```python
from build123d import *

# Parameters (mm, degrees)
SKETCH1_W               = 126
SKETCH1_H               = 126
BOSS_EXTRUDE1_DEPTH     = 5
SKETCH3_R               = 12.5
BOSS_EXTRUDE2_DEPTH     = 7.5
SKETCH4_R               = 3.45
CUT_EXTRUDE1_DEPTH      = 11.5
SKETCH6_R               = 3
CUT_EXTRUDE2_DEPTH      = 179.628805068
CHAMFER1_SIZE           = 10
CHAMFER1_SIZE_2         = 7.26542528
CUT_EXTRUDE3_DEPTH      = 179.348675353
CUT_EXTRUDE3_DEPTH_BACK = 179.348675353


with BuildPart() as part:
    # Sketch1 → Boss-Extrude1 (new body)
    with BuildSketch(Plane(origin=(0, 0, 0), x_dir=(1, 0, 0), z_dir=(0, 1, 0))):
        with Locations((63, 63)):
            Rectangle(SKETCH1_W, SKETCH1_H)
    extrude(amount=BOSS_EXTRUDE1_DEPTH)

    # Sketch3 → Boss-Extrude2 (add)
    with BuildSketch(Plane(origin=(0, 5, 0), x_dir=(1, 0, 0), z_dir=(0, 1, 0))):
        with Locations(Location((108.6, 108.6, 0), (0, 0, 90))):
            Circle(SKETCH3_R)
    extrude(amount=BOSS_EXTRUDE2_DEPTH)

    # Sketch4 → Cut-Extrude1 (cut)
    with BuildSketch(Plane.XZ):
        with Locations(Location((108.6, -108.6, 0), (0, 0, 270))):
            Circle(SKETCH4_R)
    extrude(amount=-CUT_EXTRUDE1_DEPTH, mode=Mode.SUBTRACT)

    # Sketch6 → Cut-Extrude2 (cut, through all)
    with BuildSketch(Plane(origin=(0, 12.5, 0), x_dir=(1, 0, 0), z_dir=(0, 1, 0))):
        with Locations(Location((108.6, 108.6, 0), (0, 0, 270))):
            Circle(SKETCH6_R)
    extrude(amount=-CUT_EXTRUDE2_DEPTH, mode=Mode.SUBTRACT)

    # Chamfer1
    # the kernel refuses this chamfer: 10, 7.26542528 mm, written as the material it takes off along each edge
    with BuildSketch(Plane(origin=(108.6, 12.5, -108.6), x_dir=(0, 0, -1), z_dir=(1, 0, 0))) as chamfer1_piece_1_section:
        Polygon((12.5, -CHAMFER1_SIZE), (12.5 - CHAMFER1_SIZE_2, 0), (12.5, 0), align=None)
    chamfer1_piece_1 = revolve(axis=Axis((108.6, 12.5, -108.6), (0, 1, 0)), mode=Mode.PRIVATE)
    chamfer1_piece_1 = split(chamfer1_piece_1, bisect_by=Plane(origin=(108.6, 5, -100.650989912), z_dir=(0, 1, 0)), keep=Keep.TOP, mode=Mode.PRIVATE)
    add(chamfer1_piece_1, mode=Mode.SUBTRACT)

    # Sketch7 → Cut-Extrude3 (cut, two sides: drawn at the far end of the back side and taken through both)
    with BuildSketch(Plane(origin=(0, 5, 0), x_dir=(1, 0, 0), z_dir=(0, 1, 0)).offset(-CUT_EXTRUDE3_DEPTH_BACK)):
        Polygon((70, 66.5), (89.5, 86), (109, 66.5), (89.5, 47), align=None)
        Polygon((63, 73.5), (82.5, 93), (63, 112.5), (43.5, 93), align=None)
        Polygon((56, 66.5), (36.5, 86), (17, 66.5), (36.5, 47), align=None)
        Polygon((63, 59.5), (43.5, 40), (63, 20.5), (82.5, 40), align=None)
    extrude(amount=CUT_EXTRUDE3_DEPTH + CUT_EXTRUDE3_DEPTH_BACK, mode=Mode.SUBTRACT)


solid = part.part
```
The model under review builds one solid part; all positions refer to its coordinate system, in mm. A direction names the side the tool comes from. Round coordinates to 2 decimals unless told otherwise and drop trailing zeros. Loops run counter-clockwise (first coordinate to the right, second up) from the corner with the lowest first, then second, coordinate; pieces in that order, holes last. Notation, with made-up numbers: (53.25, 8.25) -> (88.25, 8.25) arc R6 ccw to (88.25, 17.25) -> close; hole circle Ø3 at (15, -31.75). An arc over 180 degrees is marked (long way). Answer as a JSON object with one key per item and string values. Group by question number.
1) For pin 1 Ø1.5 at (x, z) = (91, -49) entering from +Y, flat-tipped, find the tip position at first contact; note if it passes through.
2) For line 1 (Z direction, x = 46, y = 2.25); line 2 (Y direction, x = 111.5, z = -35); line 3 (X direction, y = 8.75, z = -108.6), list the stretches that pass through material, from the lowest coordinate up. Write a range as [from, to].
3) For faces 1 (the face through (62, 2, 0)), 2 (the face through (53.1, 2.5, -30.4)), list the 3-axis set-ups (+Z, -Z, +X, -X, +Y, -Y) from which the entire face can be reached by the end or side of a thin tool; tool diameter is ignored.
4) Mouldability with a two-part tool opening along Z and no side actions: class faces 3 (the face through (111.95, 12.14, -104.24)), 4 (the face through (111.51, 5.67, -110.45)), 5 (the face through (62, 2, -126)) as released by +Z, released by -Z, zero draft, split by the parting line, or undercut.
5) We need section A-A on x = 30. Write out the cut boundary in (y, z), then the cut area to 3 significant figures.
6) We need section B-B on z = -108.6. Write out the cut boundary in (x, y), then the cut area to 3 significant figures.
7) We need section D-D on y = 3.5. Write out the cut boundary in (x, z).
8) We need section C-C on x = 51. Write out the cut boundary in (y, z).
Result set:
{
 "1": {"pin 1": "y = 5"},
 "2": {"line 1": "[-126, -95.5], [-90.5, -76.5], [-56.5, -42.5], [-37.5, 0]", "line 2": "[0, 5]", "line 3": "[100.64, 105.15], [112.05, 116.56]"},
 "3": {"face 1": "+Z, +X, -X, +Y, -Y", "face 2": "+Y, -Y"},
 "4": {"face 3": "split by the parting line", "face 4": "undercut", "face 5": "released by -Z"},
 "5": {"outline": "(0, -126) -> (5, -126) -> (5, -79.5) -> (0, -79.5) -> close; (0, -53.5) -> (5, -53.5) -> (5, 0) -> (0, 0) -> close", "area": "500 mm²"},
 "6": {"outline": "(0, 0) -> (59.1, 0) -> (59.1, 5) -> (0, 5) -> close; (66.9, 0) -> (105.15, 0) -> (105.15, 11.5) -> (105.6, 11.5) -> (105.6, 12.5) -> (103.37, 12.5) -> (97.92, 5) -> (66.9, 5) -> close; (111.6, 11.5) -> (112.05, 11.5) -> (112.05, 0) -> (126, 0) -> (126, 5) -> (119.28, 5) -> (113.83, 12.5) -> (111.6, 12.5) -> close", "area": "625 mm²"},
 "7": {"outline": "(0, -126) -> (126, -126) -> (126, 0) -> (0, 0) -> close; hole (17, -66.5) -> (36.5, -86) -> (56, -66.5) -> (36.5, -47) -> close; hole (43.5, -93) -> (63, -112.5) -> (82.5, -93) -> (63, -73.5) -> close; hole (43.5, -40) -> (63, -59.5) -> (82.5, -40) -> (63, -20.5) -> close; hole (70, -66.5) -> (89.5, -86) -> (109, -66.5) -> (89.5, -47) -> close; hole circle Ø6.9 at (108.6, -108.6)"},
 "8": {"outline": "(0, -126) -> (5, -126) -> (5, -100.5) -> (0, -100.5) -> close; (0, -85.5) -> (5, -85.5) -> (5, -71.5) -> (0, -71.5) -> close; (0, -61.5) -> (5, -61.5) -> (5, -47.5) -> (0, -47.5) -> close; (0, -32.5) -> (5, -32.5) -> (5, 0) -> (0, 0) -> close"}
}
